Source: CAD feature listing. Evaluate the final solid. Frame: model axes, mm. Give positions to 0.01 mm unless a question says otherwise; leave off trailing zeros. Order: outer loops, then holes, each group sorted by start corner. A loop starts at its lowest first (then second) coordinate and runs counter-clockwise, first axis right, second up. Notation, with made-up numbers: (41, 44.25) - (63, 44.25) arc R8 ccw to (63, 53.25) - close; hole circle Ø8 at (23, 55). An arc over 180 degrees is marked (long way). Answer as CSV lines item,"result".
```python
from build123d import *

# Parameters (mm, degrees)
SKETCH1_W               = 510
SKETCH1_H               = 76.2
BOSS_EXTRUDE1_DEPTH     = 3.175
SKETCH2_W               = 26
SKETCH2_H               = 32
CUT_EXTRUDE1_DEPTH      = 258.850132102
F_1_4_CLEARANCE_HOLE1_D = 6.5278
DRAFT1_ANGLE            = 10
FILLET1_R               = 12
CHAMFER1_SIZE           = 6


with BuildPart() as part:
    # Sketch1 → Boss-Extrude1 (new body)
    with BuildSketch(Plane.XY):
        Rectangle(SKETCH1_W, SKETCH1_H)
    extrude(amount=BOSS_EXTRUDE1_DEPTH)

    # Sketch2 → Cut-Extrude1 (cut, through all)
    with BuildSketch(Plane.XY.offset(3.175)):
        with Locations((121.62, -22.1)):
            Rectangle(SKETCH2_W, SKETCH2_H)
        with Locations((-121.62, -22.1)):
            Rectangle(SKETCH2_W, SKETCH2_H)
    extrude(amount=-CUT_EXTRUDE1_DEPTH, mode=Mode.SUBTRACT)

    # 1/4 Clearance Hole1 (through all)
    with Locations(Plane.XY.offset(3.175)):
        with Locations((-131.975, 13.9), (-111.265, 13.9), (111.265, 13.9), (131.975, 13.9)):
            Hole(F_1_4_CLEARANCE_HOLE1_D / 2)

    # Draft1
    draft1_faces = [part.faces().sort_by_distance(p)[0] for p in [
        (255, 0, 1.5875),
        (-255, 0, 1.5875),
    ]]
    draft(draft1_faces, Plane(origin=(255, 38.1, 3.175), x_dir=(1, 0, 0), z_dir=(0, 1, 0)), DRAFT1_ANGLE)

    # Fillet1
    fillet1_edges = [part.edges().sort_by_distance(p)[0] for p in [
        (-268.43611593, -38.1, 1.5875),
        (-255, 38.1, 1.5875),
        (255, 38.1, 1.5875),
        (268.43611593, -38.1, 1.5875),
    ]]
    fillet(fillet1_edges, radius=FILLET1_R)

    # Chamfer1
    chamfer1_edges = [part.edges().sort_by_distance(p)[0] for p in [
        (-134.62, -38.1, 1.5875),
        (134.62, -38.1, 1.5875),
        (108.62, -38.1, 1.5875),
        (-108.62, -38.1, 1.5875),
    ]]
    chamfer(chamfer1_edges, length=CHAMFER1_SIZE)


solid = part.part
```
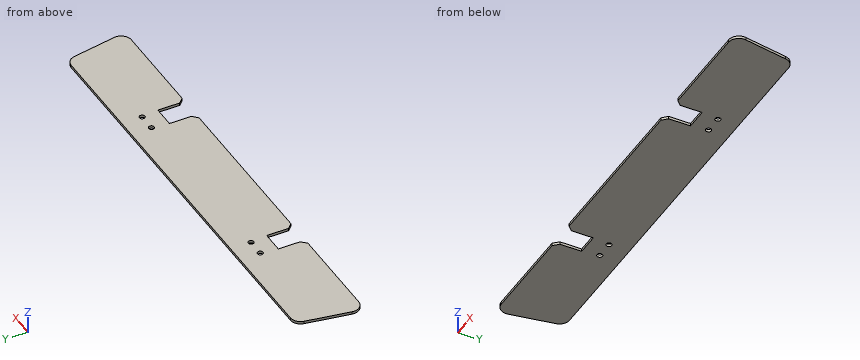
(1) Contact query for flat-ended pins moving along their axis: pin 1 (10 mm diameter, centred on x = 206.5, y = 9.5, fed in from -Z); pin 2 (1.6 mm diameter, centred on y = -22.5, z = 1, fed in from +X); pin 3 (1 mm diameter, centred on x = -121, z = 2, fed in from -Y); pin 4 (6 mm diameter, centred on x = 131.975, y = 13.9, fed in from -Z). Output: stop coordinate, or through.
Completed:
pin 1,"z = 0"
pin 2,"x = 265.83"
pin 3,"y = -6.1"
pin 4,"through"
(2) Cut plane B-B (y = 21.5). Return loops of the section in (x, z) (3 decimals).
Completed:
outline,"(-257.927, 0) - (257.927, 0) - (257.927, 3.175) - (-257.927, 3.175) - close"
(3) Ray query, line 1 (X direction, y = -26.5, z = 3); line 2 (X direction, y = -21.5, z = 2.3); line 3 (Y direction, x = 127.5, z = 2.4). Return the intervals inside material, ascending. Write a range as from..to.
Completed:
line 1,"-266.13..-134.62, -108.62..108.62, 134.62..266.13"
line 2,"-265.51..-134.62, -108.62..108.62, 134.62..265.51"
line 3,"-6.1..38.1"
(4) Cut plane A-A (z = 0.5). Return loops of the section in (x, y) (1 decimal).
Completed:
outline,"(-266, -24) arc R12 ccw to (-254.1, -38.1) - (-140.6, -38.1) - (-134.6, -32.1) - (-134.6, -6.1) - (-108.6, -6.1) - (-108.6, -32.1) - (-102.6, -38.1) - (102.6, -38.1) - (108.6, -32.1) - (108.6, -6.1) - (134.6, -6.1) - (134.6, -32.1) - (140.6, -38.1) - (254.1, -38.1) arc R12 ccw to (266, -24) - (256.7, 28.2) arc R12 ccw to (244.9, 38.1) - (-244.9, 38.1) arc R12 ccw to (-256.7, 28.2) - close; hole circle Ø6.5 at (-132, 13.9); hole circle Ø6.5 at (-111.3, 13.9); hole circle Ø6.5 at (111.3, 13.9); hole circle Ø6.5 at (132, 13.9)"
